from build123d import *

# Parameters (mm, degrees)
EXTRUDE1_START = 25.4
SKETCH1_R      = 7.9375
EXTRUDE1_DEPTH = 25.4
SKETCH2_R      = 13.335
EXTRUDE3_DEPTH = 73.025


with BuildPart() as part:
    # Sketch1 → Extrude1 (new body)
    with BuildSketch(Plane.XY.offset(EXTRUDE1_START)):
        with BuildLine():
            Line((-10.290233655, -7.443190936), (-31.75, 22.225))
            Line((-31.75, 22.225), (31.75, 22.225))
            Line((31.75, 22.225), (10.290233655, -7.443190936))
            ThreePointArc((10.290233655, -7.443190936), (0, -12.7), (-10.290233655, -7.443190936))
        make_face()
        Circle(SKETCH1_R, mode=Mode.SUBTRACT)
    extrude(amount=-EXTRUDE1_DEPTH)

    # Sketch2 → Extrude3 (cut, symmetric)
    with BuildSketch(Plane(origin=(0, 0, 0), x_dir=(0, 0, -1), z_dir=(1, 0, 0))):
        with Locations((-12.7, 22.225)):
            Circle(SKETCH2_R)
    extrude(amount=EXTRUDE3_DEPTH, both=True, mode=Mode.SUBTRACT)


solid = part.part
Verification items for the finished model (mm, model axes). Give positions to 0.01 mm unless a question says otherwise; leave off trailing zeros. Write each loop counter-clockwise with the first axis right and the second up, starting at its lowest first coordinate (ties: lowest second). Pieces come first, ordered by that corner, then holes. Notation, with made-up numbers: M -21.5,89 L 34.5,89 A15 ccw 34.5,107 Z; hole C 68,58 d5. An arc over 180 degrees is marked long. Put each result on its own line as item: value. Start each with the question number.
1. Go/stop test with flat-tipped pins: pin 1 Ø2 at (x, z) = (-2, 13) entering from +Y; pin 2 Ø8 at (x, z) = (2, 14) entering from -Y; pin 3 Ø2 at (y, z) = (9, 3.5) entering from -X; pin 4 Ø8 at (y, z) = (-5, 20) entering from -X. Record where each tip stops, or that it passes through.
2. Section check A-A (x = -2). Record the cut outline in (y, z) (3 decimals), and give its area (3 significant figures).
3. Section check D-D (x = -21). Record the cut outline in (y, z) (3 decimals), and give its area (3 significant figures).
4. Scan lines: line 1 along X through (y, z) = (-4, 7.5); line 2 along Z through (x, y) = (22, 16); line 3 along X through (y, z) = (-5, 19.75). Record each from-to range of solid material in increasing order. Write a range as [from, to].
5. Draft check along Z on faces 1 (the face through (0, 10, 0)), 2 (the face through (17.62, 2.69, 12.88)), 3 (the face through (0.403, 8.892, 12.935)). Enter one of: +Z half, -Z half, draft (parallel to the pull), parting line (faces both ways), or undercut.
6. Section check C-C (z = 6). Record the cut outline in (x, y) (1 decimal), and give its area (3 significant figures).
7. Section check B-B (y = 0). Record the cut outline in (x, z), and give its area (3 significant figures).
Answer list:
1. pin 1: y = 8.95
1. pin 2: y = -12.7
1. pin 3: x = -22.91
1. pin 4: x = -14.95
2. outline: M -12.542,0 L -7.681,0 L -7.681,25.4 L -12.542,25.4 Z; M 7.681,0 L 18.159,0 A13.335 cw 18.159,25.4 L 7.681,25.4 Z
2. area: 217 mm2
3. outline: M 7.363,0 L 18.159,0 A13.335 cw 18.159,25.4 L 7.363,25.4 Z
3. area: 102 mm2
4. line 1: [-12.78, -6.86], [6.86, 12.78]
4. line 2: [0, 0.91], [24.49, 25.4]
4. line 3: [-12.06, -6.16], [6.16, 12.06]
5. face 1: -Z half
5. face 2: draft
5. face 3: undercut
6. outline: M -23.4,10.7 L -10.3,-7.4 A12.7 ccw 10.3,-7.4 L 23.4,10.7 Z; hole C 0,0 d15.9
6. area: 489 mm2
7. outline: M -15.67,0 L -7.94,0 L -7.94,25.4 L -15.67,25.4 Z; M 7.94,0 L 15.67,0 L 15.67,25.4 L 7.94,25.4 Z
7. area: 393 mm2
